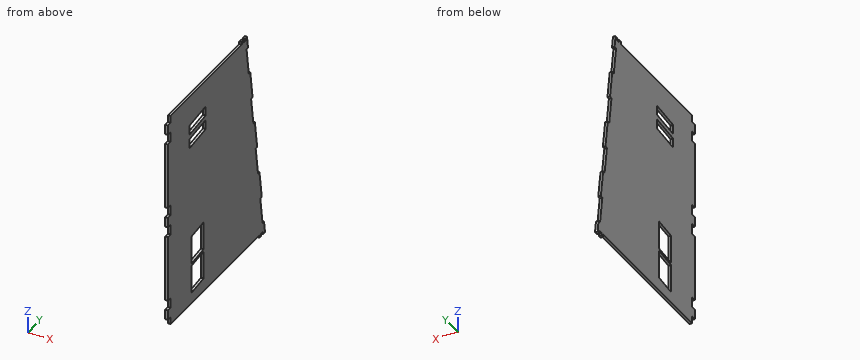
```python
from build123d import *

# Parameters (mm, degrees)
BOSS_EXTRUDE1_DEPTH = 2.7


with BuildPart() as part:
    # Sketch1 → Boss-Extrude1 (new body)
    with BuildSketch(Plane(origin=(0, 0, 0), x_dir=(0, 0, -1), z_dir=(1, 0, 0))):
        Polygon((-107.013333333, -114.8), (-96.506666667, -114.8), (-96.506666667, -109.8), (-86, -109.8), (-86, -114.8), (-16, -114.8), (-16, -109.8), (-5.333333333, -109.8), (-5.333333333, -114.8), (5.333333333, -114.8), (5.333333333, -109.8), (16, -109.8), (16, -114.8), (86, -114.8), (86, -109.8), (96.506666667, -109.8), (96.506666667, -114.8), (107.013333333, -114.8), (107.013333333, -109.8), (114.49, -109.8), (114.5, 54.7), (117.2, 54.7), (117.2, 58.033333333), (114.5, 58.033333333), (114.5, 61.366666667), (117.2, 61.366666667), (117.2, 64.7), (114.5, 64.7), (104.599212181, 63.294866357), (104.978598264, 60.621653646), (75.09310907, 56.380263258), (74.713722986, 59.05347597), (44.828233792, 54.812085582), (45.207619875, 52.138872871), (15.322130681, 47.897482483), (14.942744597, 50.570695194), (-14.942744597, 46.329304806), (-14.563358514, 43.656092095), (-44.448847708, 39.414701707), (-44.828233792, 42.087914418), (-74.713722986, 37.84652403), (-74.334336903, 35.173311319), (-104.219826097, 30.931920931), (-104.599212181, 33.605133643), (-114.5, 32.2), (-117.2, 32.2), (-117.2, 28.866666667), (-114.5, 28.866666667), (-114.5, 25.533333333), (-117.2, 25.533333333), (-117.2, 22.2), (-114.5, 22.2), (-114.5, -109.8), (-107.013333333, -109.8), align=None)
        Polygon((100.78, -48.8), (71.08, -48.8), (73.58, -70.8), (100.78, -70.8), (103.28, -70.8), align=None, mode=Mode.SUBTRACT)
        Polygon((68.58, -48.8), (71.08, -70.8), (41.38, -70.8), (38.88, -48.8), (41.38, -48.8), align=None, mode=Mode.SUBTRACT)
        Polygon((-72.910909091, -74.8), (-76.32, -44.8), (-86.32, -44.8), (-82.910909091, -74.8), align=None, mode=Mode.SUBTRACT)
        Polygon((-67.910909091, -74.8), (-71.32, -44.8), (-61.32, -44.8), (-57.910909091, -74.8), align=None, mode=Mode.SUBTRACT)
    extrude(amount=BOSS_EXTRUDE1_DEPTH)


solid = part.part
```
Here's how the part is built. I have some questions about the finished solid (model axes, mm). Coordinates: 2 decimals unless noted, no trailing zeros. Order: outer loops, then holes, each group sorted by start corner. A loop starts at its lowest first (then second) coordinate and runs counter-clockwise, first axis right, second up. Notation, with made-up numbers: (17.25, -7.5) - (76.25, -7.5) arc R16 cw to (76.25, 6.5) - close; hole circle Ø7 at (19, 7.5). An arc over 180 degrees is marked (long way). One line per question, with ' | ' between items.
(1) Suppose I cut it at D-D on z = 100. List the corners of the cut face in (x, y) for me.
Report:
outline: (0, -114.8) - (2.7, -114.8) - (2.7, 31.53) - (0, 31.53) - close
(2) Suppose I cut it at C-C on y = 0. List the corners of the cut face in (x, z) for me, and give its area (3 significant figures).
Report:
outline: (0, -114.5) - (2.7, -114.5) - (2.7, 114.5) - (0, 114.5) - close | area: 618 mm2
(3) Will these pins go through, and if not, where does the flat tip stop? pin 1 (1.4 mm diameter, centred on x = 2, y = 26.5, fed in from +Z); pin 2 (0.8 mm diameter, centred on x = 1, z = 115.5, fed in from +Y); pin 3 (1.4 mm diameter, centred on x = 0.5, z = 80, fed in from +Y).
Report:
pin 1: stops at z = 114.5 | pin 2: stops at y = 32.2 | pin 3: stops at y = 34.47
(4) Suppose I cut it at B-B on x = 1.75. State how many separate pieces and enclosed holes the cut face has, and give its area (3 significant figures).
Report:
separate pieces: 1 | enclosed holes: 4 | area: 34,900 mm2
(5) Suppose I cut it at A-A on z = -60. List the corners of the cut face in (x, y) for me.
Report:
outline: (0, -114.8) - (2.7, -114.8) - (2.7, -70.8) - (0, -70.8) - close; (0, -48.8) - (2.7, -48.8) - (2.7, 56.97) - (0, 56.97) - close
(6) If I drill on L1, parallel to Z at x = 1.3, y = -62; L2, parallel to Z at x = 1.35, y = -50.5; L3, parallel to Z at x = 1.35, y = -45.5, over which ranges is the centre line in solid material (lowest first)?
Report:
L1: z = -114.49 to -102.28, -72.58 to -70.08, -40.38 to 59.37, 69.37 to 74.37, 84.37 to 114.5 | L2: z = -114.49 to -100.97, -71.27 to -68.77, -39.07 to 60.67, 70.67 to 75.67, 85.67 to 114.5 | L3: z = -114.49 to 61.24, 71.24 to 76.24, 86.24 to 114.5
